The figure shows three views and two pictorial views of one solid part (mm, origin at its lowest corner). Answer the questions. Coordinates: 2 decimals unless noted, no trailing zeros. Loops run counter-clockwise (first coordinate to the right, second up) from the corner with the lowest first, then second, coordinate; pieces in that order, holes last. Notation, with made-up numbers: M 20,15 L 27,15 A22 cw 27,35 Z; hole C 35,-2.75 d11. An arc over 180 degrees is marked long. Write each question's results on one line, items separated by ' | '.
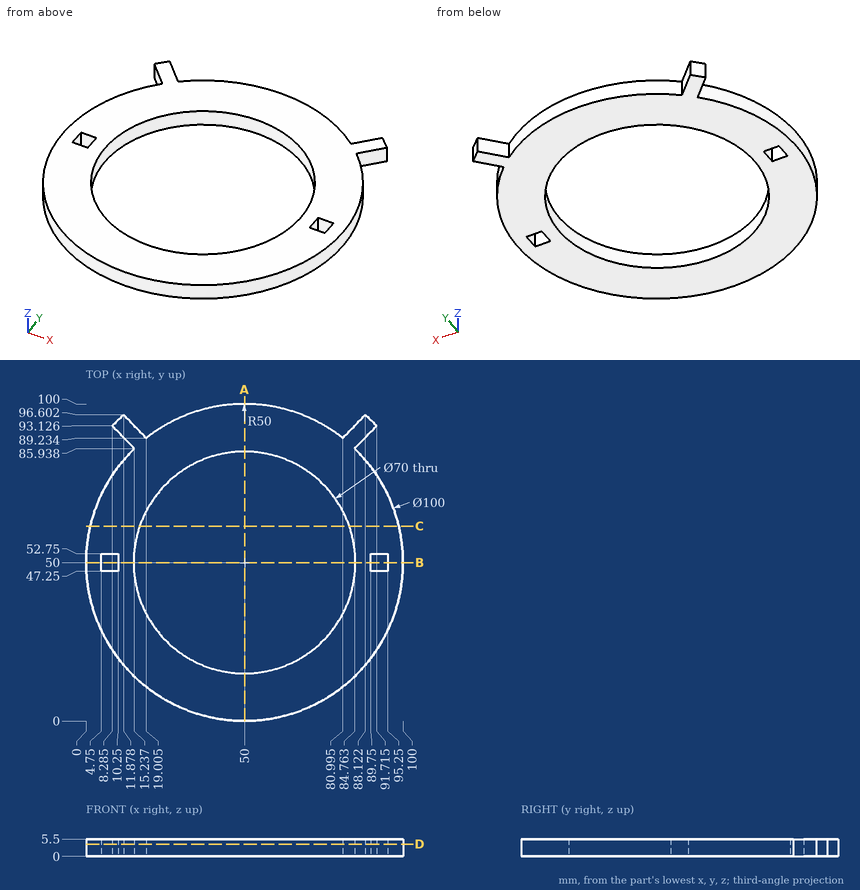
1) Find section D-D, the plane z = 3.85. Give the number of separate pieces and of enclosed holes in the cut face, and give its area (3 significant figures).
Check result:
separate pieces: 1 | enclosed holes: 3 | area: 4,050 mm^2
2) Straight lines are drawn through the part: probe 1 along Y at (x, z) = (50, 2.15); probe 2 along Y at (x, z) = (67, 3.1) (1 decimal); probe 3 along X at (y, z) = (30.5, 2.85) (1 decimal). For each, find the intervals that lie inside material, in ascending order. Write a range as [from, to].
Check result:
probe 1: [0, 15], [85, 100] | probe 2: [3, 19.4], [80.6, 97] | probe 3: [4, 20.9], [79.1, 96]
3) Find section B-B, the plane y = 50. Give the vertices of the cut face in (x, z).
Check result:
outline: M 0,0 L 4.75,0 L 4.75,5.5 L 0,5.5 Z; M 10.25,0 L 15,0 L 15,5.5 L 10.25,5.5 Z; M 85,0 L 89.75,0 L 89.75,5.5 L 85,5.5 Z; M 95.25,0 L 100,0 L 100,5.5 L 95.25,5.5 Z
4) Find section C-C, the plane y = 61.5. Give the vertices of the cut face in (x, z), and give its area (3 significant figures).
Check result:
outline: M 1.34,0 L 16.94,0 L 16.94,5.5 L 1.34,5.5 Z; M 83.06,0 L 98.66,0 L 98.66,5.5 L 83.06,5.5 Z | area: 172 mm^2
5) Given pin 1 Ø1.6 at (x, z) = (7, 3.5) entering from +Y (1 decimal); pin 2 Ø1 at (y, z) = (15.5, 1) entering from -X; pin 3 Ø1 at (y, z) = (51, 1) entering from -X, each flat-ended and moving along its own axis, determine where each tip first touches the part or whether it passes through.
Check result:
pin 1: y = 76.8 | pin 2: x = 13.34 | pin 3: x = 0
6) Find section A-A, the plane x = 50. Give the vertices of the cut face in (y, z).
Check result:
outline: M 0,0 L 15,0 L 15,5.5 L 0,5.5 Z; M 85,0 L 100,0 L 100,5.5 L 85,5.5 Z
